from build123d import *

# Parameters (mm, degrees)
EXTRUDE_1_DEPTH     = 1.2
SKETCH_2_R          = 1.375
CUT_EXTRUDE_1_DEPTH = 1.2
SKETCH_3_W          = 6
SKETCH_3_H          = 13
EXTRUDE_2_DEPTH     = 5
SKETCH_4_W          = 6
SKETCH_4_H          = 5
EXTRUDE_3_DEPTH     = 0.3
SKETCH_5_W          = 8
SKETCH_5_H          = 7
EXTRUDE_4_DEPTH     = 5.5
SKETCH_6_W          = 12
SKETCH_6_H          = 8.2
EXTRUDE_5_DEPTH     = 5.1
SKETCH_7_W          = 12
SKETCH_7_H          = 8.2
EXTRUDE_6_DEPTH     = 5.1
SKETCH_8_W          = 5.7
SKETCH_8_H          = 7.6
EXTRUDE_7_DEPTH     = 2.4
SKETCH_9_W          = 7.6
SKETCH_9_H          = 2.4
EXTRUDE_8_DEPTH     = 0.7
SKETCH_10_W         = 12
SKETCH_10_H         = 5.1
SKETCH_10_W_2       = 8
SKETCH_10_H_2       = 5.5
CUT_EXTRUDE_2_DEPTH = 0.5
SKETCH_11_W         = 51.4
SKETCH_11_H         = 5.1
EXTRUDE_9_DEPTH     = 8.5
SKETCH_12_W         = 6.2
SKETCH_12_H         = 6.2
EXTRUDE_10_DEPTH    = 3.5
SKETCH_13_R         = 1.75
EXTRUDE_11_DEPTH    = 1.5
SKETCH_14_W         = 2
SKETCH_14_H         = 2
EXTRUDE_12_DEPTH    = 1


with BuildPart() as part:
    # 草图1 → 凸台-拉伸1 (new body)
    with BuildSketch(Plane(origin=(0, 0, 0), x_dir=(1, 0, 0), z_dir=(0, 1, 0))):
        with BuildLine():
            Line((-29.5, 15), (29.5, 15))
            ThreePointArc((29.5, 15), (31.621320344, 14.121320344), (32.5, 12))
            Line((32.5, 12), (32.5, -12))
            ThreePointArc((32.5, -12), (31.621320344, -14.121320344), (29.5, -15))
            Line((29.5, -15), (-29.5, -15))
            ThreePointArc((-29.5, -15), (-31.621320344, -14.121320344), (-32.5, -12))
            Line((-32.5, -12), (-32.5, 12))
            ThreePointArc((-32.5, 12), (-31.621320344, 14.121320344), (-29.5, 15))
        make_face()
    extrude(amount=EXTRUDE_1_DEPTH)

    # 草图2 → 切除-拉伸1 (cut)
    with BuildSketch(Plane(origin=(0, 1.2, 0), x_dir=(1, 0, 0), z_dir=(0, 1, 0))):
        with Locations(Location((29, -11.5, 0), (0, 0, 270))):
            Circle(SKETCH_2_R)
        with Locations(Location((29, 11.5, 0), (0, 0, 270))):
            Circle(SKETCH_2_R)
        with Locations(Location((-29, -11.5, 0), (0, 0, 270))):
            Circle(SKETCH_2_R)
        with Locations(Location((-29, 11.5, 0), (0, 0, 270))):
            Circle(SKETCH_2_R)
    extrude(amount=-CUT_EXTRUDE_1_DEPTH, mode=Mode.SUBTRACT)

    # 草图3 → 凸台-拉伸2 (add)
    with BuildSketch(Plane(origin=(0, 1.2, 0), x_dir=(1, 0, 0), z_dir=(0, 1, 0))):
        with Locations((22.3, -8.5)):
            Rectangle(SKETCH_3_W, SKETCH_3_H)
    extrude(amount=EXTRUDE_2_DEPTH)

    # 草图4 → 凸台-拉伸3 (add)
    with BuildSketch(Plane.XY.offset(15)):
        with Locations((22.3, 3.7)):
            Rectangle(SKETCH_4_W, SKETCH_4_H)
    extrude(amount=EXTRUDE_3_DEPTH)

    # 草图5 → 凸台-拉伸4 (add)
    with BuildSketch(Plane(origin=(0, 1.2, 0), x_dir=(1, 0, 0), z_dir=(0, 1, 0))):
        with Locations((5.6, -11.5)):
            Rectangle(SKETCH_5_W, SKETCH_5_H)
    extrude(amount=EXTRUDE_4_DEPTH)

    # 草图6 → 凸台-拉伸5 (add)
    with BuildSketch(Plane(origin=(0, 1.2, 0), x_dir=(1, 0, 0), z_dir=(0, 1, 0))):
        with Locations((-5.9, -10.9)):
            Rectangle(SKETCH_6_W, SKETCH_6_H)
    extrude(amount=EXTRUDE_5_DEPTH)

    # 草图7 → 凸台-拉伸6 (add)
    with BuildSketch(Plane(origin=(0, 1.2, 0), x_dir=(1, 0, 0), z_dir=(0, 1, 0))):
        with Locations((-19.45, -10.9)):
            Rectangle(SKETCH_7_W, SKETCH_7_H)
    extrude(amount=EXTRUDE_6_DEPTH)

    # 草图8 → 凸台-拉伸7 (add)
    with BuildSketch(Plane(origin=(0, 1.2, 0), x_dir=(1, 0, 0), z_dir=(0, 1, 0))):
        with Locations((-29.65, -1.5)):
            Rectangle(SKETCH_8_W, SKETCH_8_H)
    extrude(amount=EXTRUDE_7_DEPTH)

    # 草图9 → 凸台-拉伸8 (add)
    with BuildSketch(Plane.ZY.offset(32.5)):
        with Locations((1.5, 2.4)):
            Rectangle(SKETCH_9_W, SKETCH_9_H)
    extrude(amount=EXTRUDE_8_DEPTH)

    # 草图10 → 切除-拉伸2 (cut)
    with BuildSketch(Plane.XY.offset(15)):
        with Locations((-19.45, 3.75)):
            Rectangle(SKETCH_10_W, SKETCH_10_H)
        with Locations((-5.9, 3.75)):
            Rectangle(SKETCH_10_W, SKETCH_10_H)
        with Locations((5.6, 3.95)):
            Rectangle(SKETCH_10_W_2, SKETCH_10_H_2)
    extrude(amount=-CUT_EXTRUDE_2_DEPTH, mode=Mode.SUBTRACT)

    # 草图11 → 凸台-拉伸9 (add)
    with BuildSketch(Plane.XZ):
        with Locations((-0.05, -11.55)):
            Rectangle(SKETCH_11_W, SKETCH_11_H)
    extrude(amount=EXTRUDE_9_DEPTH)

    # 草图12 → 凸台-拉伸10 (add)
    with BuildSketch(Plane(origin=(0, 1.2, 0), x_dir=(1, 0, 0), z_dir=(0, 1, 0))):
        with Locations((-16.2, 2.6)):
            Rectangle(SKETCH_12_W, SKETCH_12_H)
    extrude(amount=EXTRUDE_10_DEPTH)

    # 草图13 → 凸台-拉伸11 (add)
    with BuildSketch(Plane(origin=(0, 4.7, 0), x_dir=(1, 0, 0), z_dir=(0, 1, 0))):
        with Locations(Location((-16.2, 2.6, 0), (0, 0, 270))):
            Circle(SKETCH_13_R)
    extrude(amount=EXTRUDE_11_DEPTH)

    # 草图14 → 凸台-拉伸12 (add)
    with BuildSketch(Plane(origin=(0, 1.2, 0), x_dir=(1, 0, 0), z_dir=(0, 1, 0))):
        with Locations((3.2, 3.22)):
            Rectangle(SKETCH_14_W, SKETCH_14_H)
        with Locations((0, 3.22)):
            Rectangle(SKETCH_14_W, SKETCH_14_H)
        with Locations((-3.2, 3.22)):
            Rectangle(SKETCH_14_W, SKETCH_14_H)
    extrude(amount=EXTRUDE_12_DEPTH)


solid = part.part
Read the model definition and answer for the solid it produces. Units are mm, in the model's axes. A direction names the side the tool comes from. Give positions to 0.01 mm unless a question says otherwise; leave off trailing zeros. Loops run counter-clockwise (first coordinate to the right, second up) from the corner with the lowest first, then second, coordinate; pieces in that order, holes last. Notation, with made-up numbers: (40.5, 71) -> (52.5, 71) arc R20 ccw to (52.5, 103) -> close; hole circle Ø8 at (-0.5, 19.5). An arc over 180 degrees is marked (long way). Answer as CSV lines item,"result".
Item 1: Each of these flat-tipped pins is pushed along its axis until it touches: pin 1 (1.9 mm diameter, centred on x = -17, z = -2.5, fed in from +Y); pin 2 (2.5 mm diameter, centred on y = 4.5, z = 8.5, fed in from +X); pin 3 (1.8 mm diameter, centred on x = -17.5, y = 3, fed in from -Z). Where does it stop, or does it pass through?
Returned:
pin 1,"stops at y = 6.2"
pin 2,"stops at x = 25.3"
pin 3,"stops at z = -5.7"
Item 2: Find section A-A on x = 11. Give the vertices of the cut face in (y, z), plus the area to 4 significant figures.
Returned:
outline,"(-8.5, -14.1) -> (0, -14.1) -> (0, -15) -> (1.2, -15) -> (1.2, 15) -> (0, 15) -> (0, -9) -> (-8.5, -9) -> close"
area,"79.35 mm²"
Item 3: Find section C-C on y = -1.75. Give the vertices of the cut face in (x, z), plus the area to 3 significant figures.
Returned:
outline,"(-25.75, -14.1) -> (25.65, -14.1) -> (25.65, -9) -> (-25.75, -9) -> close"
area,"262 mm²"
Item 4: Find section D-D on x = -16.2. Give the vertices of the cut face in (y, z), plus the area to 3 significant figures.
Returned:
outline,"(-8.5, -14.1) -> (0, -14.1) -> (0, -15) -> (1.2, -15) -> (1.2, -5.7) -> (4.7, -5.7) -> (4.7, -4.35) -> (6.2, -4.35) -> (6.2, -0.85) -> (4.7, -0.85) -> (4.7, 0.5) -> (1.2, 0.5) -> (1.2, 6.8) -> (6.3, 6.8) -> (6.3, 14.5) -> (1.2, 14.5) -> (1.2, 15) -> (0, 15) -> (0, -9) -> (-8.5, -9) -> close"
area,"146 mm²"
Item 5: Determine the mould class of faces 4 (the face through (-6, 4, 6.8)), 5 (the face through (-26.8, 2, 2)), 6 (the face through (25.65, -4, -12)) for opening direction X: +X half, -X half, draft (parallel to the pull), parting line (faces both ways), or undercut.
Returned:
face 4,"draft"
face 5,"undercut"
face 6,"+X half"
Item 6: For faces 1 (the face through (-3, 2.2, -3)), 2 (the face through (-18, 4.7, -4)), 3 (the face through (-20, 4, 14.5)), determine the directions among +Z, -Z, +X, -X, +Y, -Y from which every point of the face is accessible in a straight line to the end or side of a thin tool.
Returned:
face 1,"-Z, +X, +Y"
face 2,"+Y"
face 3,"+Z, -X, +Y"
Item 7: Consider line 1 (X direction, y = 0.45, z = -11.5) (3 decimals); line 2 (Z direction, x = 23, y = -0.75); line 3 (Y direction, x = 16, z = -11.5). Determine where each line is inside the solid, lowest interval first. Write a range as [from, to].
Returned:
line 1,"x = [-32.5, -30.375], [-27.625, 27.625], [30.375, 32.5]"
line 2,"z = [-14.1, -9]"
line 3,"y = [-8.5, 1.2]"
Item 8: Find section B-B on z = 3. Give the vertices of the cut face in (x, y).
Returned:
outline,"(-33.2, 1.2) -> (-32.5, 1.2) -> (-32.5, 0) -> (32.5, 0) -> (32.5, 1.2) -> (25.3, 1.2) -> (25.3, 6.2) -> (19.3, 6.2) -> (19.3, 1.2) -> (-26.8, 1.2) -> (-26.8, 3.6) -> (-33.2, 3.6) -> close"
